The model under review builds one solid part; all positions refer to its coordinate system, in mm. A direction names the side the tool comes from. Give positions to 0.01 mm unless a question says otherwise; leave off trailing zeros. Order: outer loops, then holes, each group sorted by start corner. A loop starts at its lowest first (then second) coordinate and runs counter-clockwise, first axis right, second up. Notation, with made-up numbers: (20.25, -1.75) - (79.25, -1.75) arc R8 ccw to (79.25, 2.25) - close; hole circle Ø9 at (-23, -36). An arc over 180 degrees is marked (long way). Write item = value, one per line. Start each with the question number.
1. We need section D-D, the plane x = -6.25. Give the boundary of the cut face in (y, z), and give its area (3 significant figures).
2. Machinability: for faces 1 (the flat face through (-5, 0, 5.6)), 2 (the flat face through (1, 10, 2.5)), 3 (the flat face through (7.5, 0, 5)), which of the approach directions +Z, -Z, +X, -X, +Y, -Y give a long, thin tool a straight path to every point of the face, cutting with its end or side? Answer none if there is none.
3. For P1, Ø4, axis at x = 0, y = 11.5, coming from the -Z side; P2, Ø4.5, axis at x = -1.5, y = -11, coming from the -Z side; P3, Ø2.5, axis at y = 3.5, z = 8, coming from the -X side; P4, Ø2.5, axis at x = 0, y = -11.5, coming from the +Z side, all flat-tipped, find the tip position at first contact; note any pin that passes through.
4. We need section B-B, the plane y = 0. Give the boundary of the cut face in (x, z), and give its area (3 significant figures).
5. Wall thickness on probe 1 along Y at (x, z) = (1.25, 8); probe 2 along Y at (x, z) = (0, 6.25); probe 3 along X at (y, z) = (-11.5, 7.75): over which ranges is each line inside the solid? List them lowest first.
6. Mouldability with a two-part tool opening along X and no side actions: class faces 4 (the flat face through (-10, 0, 3)), 5 (the cylindrical face through (0, -10, 7)), 6 (the cylindrical face through (-8.77, 0.18, 3.82)) as pulls with the +X half, pulls with the -X half, needs draft (parallel to the pull), parting line crosses it, or undercut.
7. We need section A-A, the plane z = 1.25. Give the boundary of the cut face in (x, y), and give its area (3 significant figures).
8. We need section C-C, the plane x = 0. Give the boundary of the cut face in (y, z), and give its area (3 significant figures).
from build123d import *

# Parameters (mm, degrees)
SKETCH002_R     = 8.1
PAD001_DEPTH    = 5
SKETCH_W        = 15
SKETCH_H        = 30
PAD_DEPTH       = 12.1
SKETCH001_R     = 6.2
POCKET_DEPTH    = 15.001
SKETCH003_R     = 1.5
POCKET001_DEPTH = 12.101
POCKET002_DEPTH = 2.5
SKETCH005_W     = 30
SKETCH005_H     = 12.1
PAD002_DEPTH    = 2.5
SKETCH006_R     = 8.2
POCKET003_DEPTH = 2.5


with BuildPart() as pad001:
    # Sketch002 → Pad001 (new body, symmetric)
    with BuildSketch(Plane.YZ):
        with Locations((0, 12)):
            Circle(SKETCH002_R)
    extrude(amount=PAD001_DEPTH, both=True)


with BuildPart() as pocket003:
    # Sketch → Pad (new body)
    with BuildSketch(Plane.XY):
        Rectangle(SKETCH_W, SKETCH_H)
    extrude(amount=PAD_DEPTH)

    # Sketch001 → Pocket (cut, through all)
    with BuildSketch(Plane.YZ.offset(7.5)):
        with Locations((0, 12)):
            Circle(SKETCH001_R)
    extrude(amount=-POCKET_DEPTH, mode=Mode.SUBTRACT)

    # Cut: cut Pad001
    add(pad001.part, mode=Mode.SUBTRACT)

    # Sketch003 → Pocket001 (cut, through all)
    with BuildSketch(Plane(origin=(0, 0, 0), x_dir=(1, 0, 0), z_dir=(0, 0, -1))):
        with Locations((0, 11.5)):
            Circle(SKETCH003_R)
        with Locations((0, -11.5)):
            Circle(SKETCH003_R)
    extrude(amount=-POCKET001_DEPTH, mode=Mode.SUBTRACT)

    # Sketch004 → Pocket002 (cut)
    with BuildSketch(Plane(origin=(0, 0, 0), x_dir=(1, 0, 0), z_dir=(0, 0, -1))):
        Polygon((3.2, 11.5), (1.6, 14.271281), (-1.6, 14.271281), (-3.2, 11.5), (-1.6, 8.728719), (1.6, 8.728719), align=None)
        Polygon((1.6, -14.271281), (3.2, -11.5), (1.6, -8.728719), (-1.6, -8.728719), (-3.2, -11.5), (-1.6, -14.271281), align=None)
    extrude(amount=-POCKET002_DEPTH, mode=Mode.SUBTRACT)

    # Sketch005 → Pad002 (new body)
    with BuildSketch(Plane(origin=(-7.5, 0, 0), x_dir=(0, -1, 0), z_dir=(-1, 0, 0))):
        with Locations((0, 6.05)):
            Rectangle(SKETCH005_W, SKETCH005_H)
    extrude(amount=PAD002_DEPTH)

    # Sketch006 → Pocket003 (cut)
    with BuildSketch(Plane(origin=(-10, 0, 0), x_dir=(0, -1, 0), z_dir=(-1, 0, 0))):
        with Locations((0, 12.016602)):
            Circle(SKETCH006_R)
    extrude(amount=-POCKET003_DEPTH, mode=Mode.SUBTRACT)


solid = pocket003.part
Model answer:
q1.outline = (-15, 0) - (15, 0) - (15, 12.1) - (6.2, 12.1) arc R6.2 cw (long way) to (-6.2, 12.1) - (-15, 12.1) - close
q1.area = 301 mm2
q2.face_1 = +Z
q2.face_2 = -Z
q2.face_3 = +Z, -Z, +X, +Y, -Y
q3.P1 = 2.5
q3.P2 = 0
q3.P3 = -7.5
q3.P4 = through
q4.outline = (-10, 0) - (7.5, 0) - (7.5, 5.8) - (5, 5.8) - (5, 3.9) - (-5, 3.9) - (-5, 5.8) - (-7.5, 5.8) - (-7.5, 3.82) - (-10, 3.82) - close
q4.area = 77.5 mm2
q5.probe_1 = -15 to -12.33, -10.67 to -7.04, 7.04 to 10.67, 12.33 to 15
q5.probe_2 = -15 to -13, -10 to -5.71, 5.71 to 10, 13 to 15
q5.probe_3 = -10 to -1.5, 1.5 to 7.5
q6.face_4 = pulls with the -X half
q6.face_5 = undercut
q6.face_6 = needs draft
q7.outline = (-10, -15) - (7.5, -15) - (7.5, 15) - (-10, 15) - close; hole (-3.2, -11.5) - (-1.6, -14.27) - (1.6, -14.27) - (3.2, -11.5) - (1.6, -8.73) - (-1.6, -8.73) - close; hole (-3.2, 11.5) - (-1.6, 8.73) - (1.6, 8.73) - (3.2, 11.5) - (1.6, 14.27) - (-1.6, 14.27) - close
q7.area = 472 mm2
q8.outline = (-15, 0) - (-14.27, 0) - (-14.27, 2.5) - (-13, 2.5) - (-13, 12.1) - (-15, 12.1) - close; (-10, 2.5) - (-8.73, 2.5) - (-8.73, 0) - (8.73, 0) - (8.73, 2.5) - (10, 2.5) - (10, 12.1) - (8.1, 12.1) arc R8.1 cw (long way) to (-8.1, 12.1) - (-10, 12.1) - close; (13, 2.5) - (14.27, 2.5) - (14.27, 0) - (15, 0) - (15, 12.1) - (13, 12.1) - close
q8.area = 173 mm2
